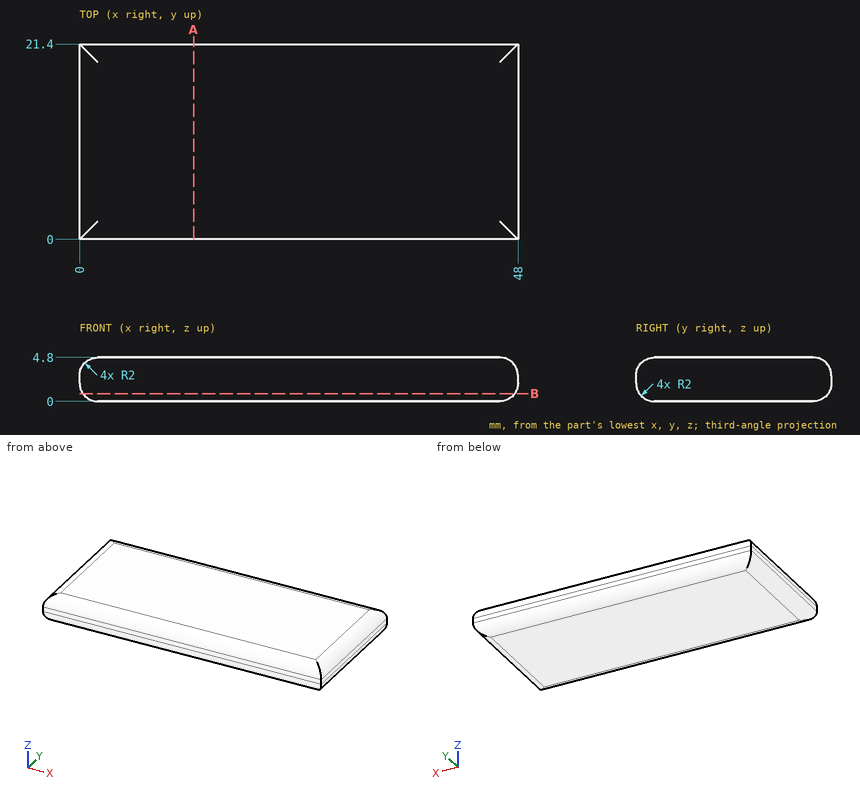
The drawing under review shows one solid part. Ordinate dimensions are in mm from its lowest x, y, z. Coordinates: 2 decimals unless noted, no trailing zeros. Order: outer loops, then holes, each group sorted by start corner. A loop starts at its lowest first (then second) coordinate and runs counter-clockwise, first axis right, second up. Notation, with made-up numbers: M 14.25,50.25 L 21.25,50.25 A19 cw 21.25,78.25 Z; hole C 57.5,-38 d9. An arc over 180 degrees is marked long. Use a Markdown table: item, result.
(1) Add section A-A (x = 12.5). Give the boundary of the cut face in (y, z), then the cut area to 3 significant figures.
Worked answers:
| item | result |
|---|---|
| outline | M 0,2 A2 ccw 2,0 L 19.4,0 A2 ccw 21.4,2 L 21.4,2.8 A2 ccw 19.4,4.8 L 2,4.8 A2 ccw 0,2.8 Z |
| area | 99.3 mm2 |
(2) Wall thickness on probe 1 along Y at (x, z) = (5, 1.8); probe 2 along X at (y, z) = (1.75, 3.4); probe 3 along X at (y, z) = (7, 1.65): over which ranges is each line inside the solid? List them lowest first.
Worked answers:
| item | result |
|---|---|
| probe 1 | y = 0.01 to 21.39 |
| probe 2 | x = 0.09 to 47.91 |
| probe 3 | x = 0.03 to 47.97 |
(3) For P1, Ø2, axis at x = 15, y = 11.5, coming from the -Z side, flat-tipped, find the tip position at first contact; note if it passes through.
Worked answers:
| item | result |
|---|---|
| P1 | stops at z = 0 |
(4) Add section B-B (z = 0.85). Give the boundary of the cut face in (x, y), then the cut area to 3 significant figures.
Worked answers:
| item | result |
|---|---|
| outline | M 0.36,0.36 L 47.64,0.36 L 47.64,21.04 L 0.36,21.04 Z |
| area | 977 mm2 |
